Part print with two shaded views. Sizes in mm from the minimum x, y, z corner. Round coordinates to 2 decimals unless told otherwise and drop trailing zeros. Write each loop counter-clockwise with the first axis right and the second up, starting at its lowest first coordinate (ties: lowest second). Pieces come first, ordered by that corner, then holes. Notation, with made-up numbers: M 14.25,-14 L 27.25,-14 A12 cw 27.25,-7 Z; hole C 4,-37 d6. An arc over 180 degrees is marked long. Use one line per item in the form item = value. Start each with the question number.
Item 1: Flat gauge pins, fed straight in: pin 1 Ø1.8 at (y, z) = (15, 3) entering from +X; pin 2 Ø3 at (y, z) = (3.5, 1.5) entering from -X; pin 3 Ø3 at (y, z) = (2.5, 3) entering from +X. Where does each tip first touch, or does it go through?
Item 2: Cut at A-A, the plane z = 3. State how many separate pieces and enclosed holes the cut face has, then the cut area to 3 significant figures.
Item 3: Cut at C-C, the plane y = 37. Give the cut face in (x, z).
Item 4: Cut at B-B, the plane x = 23. Give the cut face in (y, z), then the cut area to 3 significant figures.
Item 5: Probe L1, parallel to X at y = 62, z = 2; L2, parallel to Y at x = 65, z = 4.05; L3, parallel to X at y = 30.5, z = 0.65. List the from-to ranges inside material, lowest first.
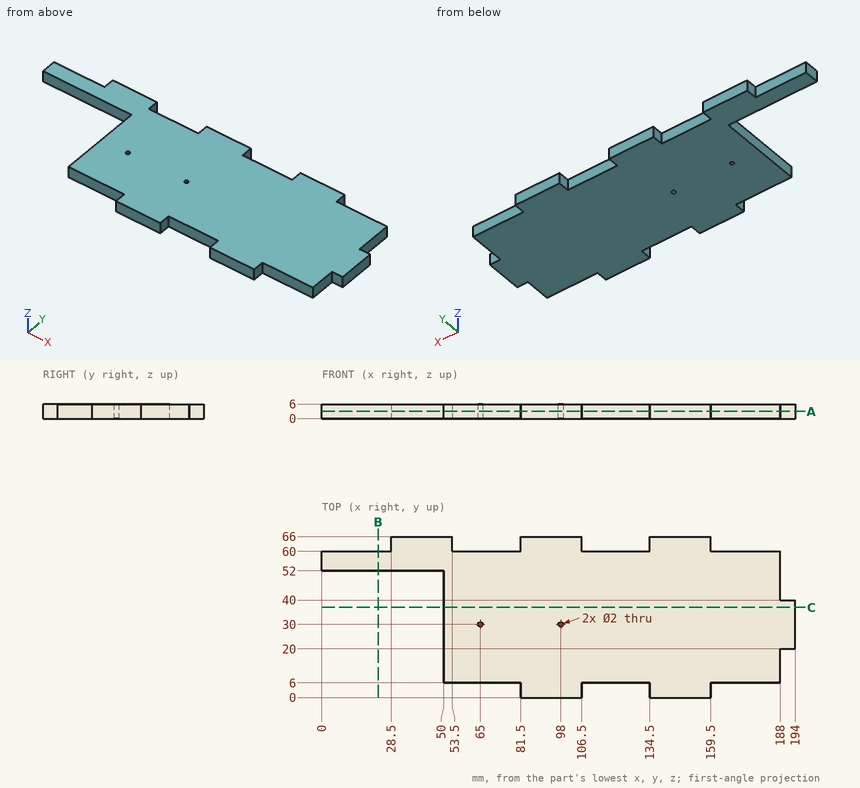
Model answer:
q1.pin_1 = 188
q1.pin_2 = 81.5
q1.pin_3 = 159.5
q2.separate_pieces = 1
q2.enclosed_holes = 2
q2.area = 8,720 mm²
q3.outline = M 50,0 L 194,0 L 194,6 L 50,6 Z
q4.outline = M 52,0 L 60,0 L 60,6 L 52,6 Z
q4.area = 48.0 mm²
q5.L1 = 28.5 to 53.5, 81.5 to 106.5, 134.5 to 159.5
q5.L2 = 6 to 29, 31 to 60
q5.L3 = 50 to 64.13, 65.87 to 97.13, 98.87 to 194
